Geometry: final body of the model. Coordinates: model frame, mm. Give positions to 0.01 mm unless a question says otherwise; leave off trailing zeros. Order: outer loops, then holes, each group sorted by start corner. A loop starts at its lowest first (then second) coordinate and runs counter-clockwise, first axis right, second up. Notation, with made-up numbers: (72.5, 56) -> (87.5, 56) arc R33 ccw to (87.5, 86) -> close; hole circle Ø1 at (26.25, 26). An arc over 180 degrees is marked (long way). One line per item, written item: value. Start each with the question number.
Autodesk Inventor part; units mm, degrees
ref_plane "YZ Plane" through (0, 0, 0) normal (1, 0, 0) x (0, 1, 0)
ref_plane "XZ Plane" through (0, 0, 0) normal (0, 1, 0) x (-1, 0, 0)
ref_plane "XY Plane" through (0, 0, 0) normal (0, 0, 1) x (1, 0, 0)
sketch "Sketch1" plane through (0, 0, 0) normal (0, 1, 0) x (-1, 0, 0)
  line L0 (0, 0) -> (30.988, 0)
  line L1 (30.988, 0) -> (30.988, -30.988)
  line L2 (30.988, -30.988) -> (0, -30.988)
  line L3 (0, -30.988) -> (0, 0)
  dimension "d0" = 30.988
  dimension "d1" = 30.988
extrude "Extrusion1" add sketch "Sketch1" along normal blind 2.54
sketch "Sketch2" plane through (0, 2.54, 0) normal (0, 1, 0) x (1, 0, 0)
  circle A0 centre (-3.556, 3.556) radius 1.778
  line L0 (0, 0) -> (0, 30.988)
  line L1 (-30.988, 0) -> (0, 0)
  circle A1 centre (-27.432, 3.556) radius 1.778
  circle A2 centre (-3.556, 27.432) radius 1.778
  circle A3 centre (-27.432, 27.432) radius 1.778
  dimension "d4" = 3.556
  dimension "d5" = 3.556
  dimension "d6" = 3.556
  dimension "d9" = 23.876
  dimension "d12" = 23.876
extrude "Extrusion2" cut sketch "Sketch2" against normal blind 2.54
chamfer "Chamfer1" distance 1.524 distance2 1.27 1 edges at (-29.21, 2.54, -3.556) measured on face at (-11.9583, 2.54, -19.0803)
chamfer "Chamfer2" distance 1.524 distance2 1.27 1 edges at (-5.334, 2.54, -3.556) measured on face at (-18.6495, 2.54, -19.4172)
chamfer "Chamfer3" distance 1.524 distance2 1.27 1 edges at (-5.334, 2.54, -27.432) measured on face at (-18.6495, 2.54, -19.4172)
chamfer "Chamfer4" distance 1.524 distance2 1.27 1 edges at (-29.21, 2.54, -27.432) measured on face at (-19.2283, 2.54, -19.2563)
fillet "Fillet1" radius 1.27 4 edges at (0, 1.27, 0) (0, 1.27, -30.988) (-30.988, 1.27, -30.988) (-30.988, 1.27, 0)
properties part number "ForeAftMountPlate" material "ABS Plastic"
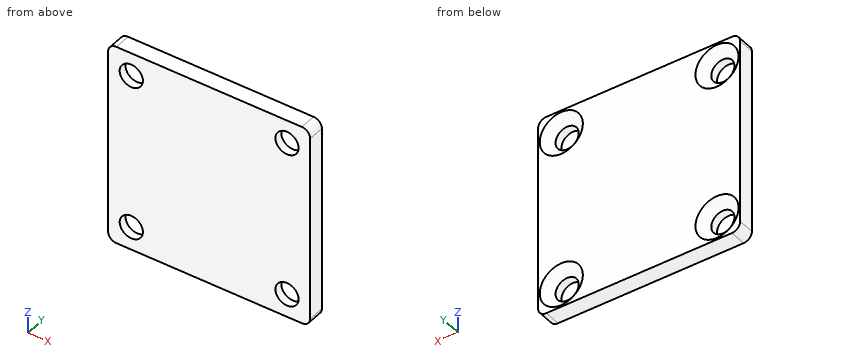
1. Cut plane B-B, the plane x = -3.5. State how many separate pieces and enclosed holes the cut face has, then the cut area to 3 significant figures.
2. Cut plane A-A, the plane y = 1.8. Return loops of the section in (x, z).
3. Material intervals for L1, parallel to Z at x = -3, y = 0.35; L2, parallel to Z at x = -3.5, y = 2.15; L3, parallel to Y at x = -2.5, z = -2, sorted ascending. Write a range as [from, to].
Answers follow:
1. separate pieces: 3
1. enclosed holes: 0
1. area: 56.8 mm²
2. outline: (-30.99, -29.72) arc R1.27 ccw to (-29.72, -30.99) -> (-1.27, -30.99) arc R1.27 ccw to (0, -29.72) -> (0, -1.27) arc R1.27 ccw to (-1.27, 0) -> (-29.72, 0) arc R1.27 ccw to (-30.99, -1.27) -> close; hole circle Ø4.83 at (-27.43, -27.43); hole circle Ø4.83 at (-27.43, -3.56); hole circle Ø4.83 at (-3.56, -27.43); hole circle Ø4.83 at (-3.56, -3.56)
3. L1: z = [-30.99, -29.12], [-25.74, -5.24], [-1.87, 0]
3. L2: z = [-30.99, -30.27], [-24.6, -6.39], [-0.72, 0]
3. L3: y = [0, 1.36]
